```python
from build123d import *

# Parameters (mm, degrees)
F0_W     = 1.70942
F0_H     = 3.175
F1_DEPTH = 6


with BuildPart() as f1:
    # F0 (on Top) → F1 (new body)
    with BuildSketch(Plane.XY):
        with BuildLine():
            Line((3.70942, 2), (-2, 2))
            Line((-2, 2), (-2, -68.675))
            ThreePointArc((-2, -68.675), (-8.35, -75.025), (-14.7, -68.675))
            Line((-14.7, -68.675), (-14.7, 138.442501))
            ThreePointArc((-14.7, 138.442501), (-8.35, 144.792501), (-2, 138.442501))
            Line((-2, 138.442501), (-2, 67.767501))
            Line((-2, 67.767501), (3.70942, 67.767501))
            Line((3.70942, 67.767501), (3.70942, 74.942501))
            Line((3.70942, 74.942501), (2, 74.942501))
            Line((2, 74.942501), (2, 87.642501))
            Line((2, 87.642501), (0, 87.642501))
            Line((0, 87.642501), (0, 138.442501))
            ThreePointArc((0, 138.442501), (-8.35, 146.792501), (-16.7, 138.442501))
            Line((-16.7, 138.442501), (-16.7, -68.675))
            ThreePointArc((-16.7, -68.675), (-8.35, -77.025), (0, -68.675))
            Line((0, -68.675), (0, -17.875))
            Line((0, -17.875), (2, -17.875))
            Line((2, -17.875), (2, -5.175))
            Line((2, -5.175), (3.70942, -5.175))
            Line((3.70942, -5.175), (3.70942, 2))
        make_face()
        with Locations((0.85471, -1.5875)):
            Rectangle(F0_W, F0_H, mode=Mode.SUBTRACT)
        with Locations((0.85471, 71.355001)):
            Rectangle(F0_W, F0_H, mode=Mode.SUBTRACT)
    extrude(amount=F1_DEPTH)


solid = f1.part
```
The listing builds one solid part. Answer for the finished solid, in the listing's coordinates (mm). A direction names the side the tool comes from. Give positions to 0.01 mm unless a question says otherwise; leave off trailing zeros. Write each loop counter-clockwise with the first axis right and the second up, starting at its lowest first coordinate (ties: lowest second). Pieces come first, ordered by that corner, then holes. Notation, with made-up numbers: (0, 19) -> (36, 19) arc R13 cw to (36, 31) -> close; hole circle Ø9 at (25.5, -22.5). An arc over 180 degrees is marked (long way). Write item = value, one per line. Start each with the question number.
1) The part is cut by section A-A, the plane x = -8.35. Determine the outline of the cut face in (y, z) (1 decimal), and give its area (3 significant figures).
2) Each of these flat-tipped pins is pushed along its axis until it touches: pin 1 (1 mm diameter, centred on y = 15.5, z = 1.5, fed in from +X); pin 2 (0.9 mm diameter, centred on x = 1, z = 2, fed in from +Y); pin 3 (0.9 mm diameter, centred on x = 3, z = 3, fed in from -Y) (3 decimals). Where does it stop, or does it pass through?
3) Straight lines are drawn through the part: line 1 along Y through (x, z) = (1.25, 2.45) (1 decimal); line 2 along X through (y, z) = (122.5, 2.4); line 3 along X through (y, z) = (-12, 2.45). For each, find the intervals that lie inside material, in ascending order.
4) Determine the mould class of faces 1 (the face through (-8.17, 146.79, 2.96)), 2 (the face through (-2, 104, 3)), 3 (the face through (-16, 35, 6)) for opening direction X: +X half, -X half, draft (parallel to the pull), parting line (faces both ways), or undercut.
5) The part is cut by section B-B, the plane z = 1.4. Count the separate pieces of the cut face and the enclosed holes in it, and give its area (3 significant figures).
6) The part is cut by section C-C, the plane y = -30.5. Determine the outline of the cut face in (x, z).
7) Which of the six approach directions +Z, -Z, +X, -X, +Y, -Y give full straight-line access (tool end or side, diameter ignored) to faces 4 (the face through (0, 113, 3)), 5 (the face through (-14.7, 33, 3)), 6 (the face through (1, 67.768, 3)), 7 (the face through (2, -12, 3))?
8) The part is cut by section D-D, the plane y = 27. Determine the outline of the cut face in (x, z), and give its area (3 significant figures).
Solutions:
q1.outline = (-77, 0) -> (-75, 0) -> (-75, 6) -> (-77, 6) -> close; (144.8, 0) -> (146.8, 0) -> (146.8, 6) -> (144.8, 6) -> close
q1.area = 24.0 mm²
q2.pin_1 = -14.7
q2.pin_2 = 87.64
q2.pin_3 = -5.175
q3.line_1 = -17.9 to -3.2, 0 to 2, 67.8 to 69.8, 72.9 to 87.6
q3.line_2 = -16.7 to -14.7, -2 to 0
q3.line_3 = -16.7 to -14.7, -2 to 2
q4.face_1 = parting line
q4.face_2 = undercut
q4.face_3 = draft
q5.separate_pieces = 1
q5.enclosed_holes = 2
q5.area = 882 mm²
q6.outline = (-16.7, 0) -> (-14.7, 0) -> (-14.7, 6) -> (-16.7, 6) -> close; (-2, 0) -> (0, 0) -> (0, 6) -> (-2, 6) -> close
q7.face_4 = +Z, -Z, +X, +Y
q7.face_5 = +Z, -Z
q7.face_6 = +Z, -Z, +X
q7.face_7 = +Z, -Z, +X, -Y
q8.outline = (-16.7, 0) -> (-14.7, 0) -> (-14.7, 6) -> (-16.7, 6) -> close
q8.area = 12.0 mm²
